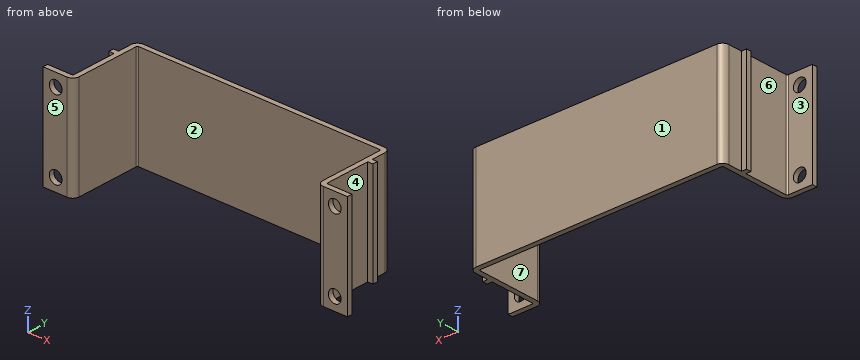
from build123d import *

# Parameters (mm, degrees)
BASE_FLANGE1_DEPTH  = 40
CUT_EXTRUDE1_REACH  = 132
SKETCH6_R           = 2.5
SKETCH7_W           = 2
SKETCH7_H           = 2
BOSS_EXTRUDE1_DEPTH = 40


# Sheet-metal steps are written as plain solids
with BuildPart() as part:
    # Sketch1 → Base-Flange1 (new body)
    with BuildSketch(Plane.XY):
        with BuildLine():
            Line((0, 0), (9.5, 0))
            ThreePointArc((9.5, 0), (9.853553391, 0.146446609), (10, 0.5))
            Line((10, 0.5), (10, 25.5))
            ThreePointArc((10, 25.5), (10.732233047, 27.267766953), (12.5, 28))
            Line((12.5, 28), (107.5, 28))
            ThreePointArc((107.5, 28), (109.267766953, 27.267766953), (110, 25.5))
            Line((110, 25.5), (110, 0.5))
            ThreePointArc((110, 0.5), (110.146446609, 0.146446609), (110.5, 0))
            Line((110.5, 0), (120, 0))
            Line((120, 0), (120, -2))
            Line((120, -2), (110.5, -2))
            ThreePointArc((110.5, -2), (108.732233047, -1.267766953), (108, 0.5))
            Line((108, 0.5), (108, 25.5))
            ThreePointArc((108, 25.5), (107.853553391, 25.853553391), (107.5, 26))
            Line((107.5, 26), (12.5, 26))
            ThreePointArc((12.5, 26), (12.146446609, 25.853553391), (12, 25.5))
            Line((12, 25.5), (12, 0.5))
            ThreePointArc((12, 0.5), (11.267766953, -1.267766953), (9.5, -2))
            Line((9.5, -2), (0, -2))
            Line((0, -2), (0, 0))
        make_face()
    extrude(amount=BASE_FLANGE1_DEPTH)

    # Sketch6 → Cut-Extrude1 (cut, up to next)
    with BuildSketch(Plane.XZ.offset(2), mode=Mode.PRIVATE) as cut_extrude1_sk1:
        with Locations(Location((5, 35, 0), (0, 0, 270))):
            Circle(SKETCH6_R)
    cut_extrude1_tool1 = extrude(cut_extrude1_sk1.sketch, amount=-CUT_EXTRUDE1_REACH, mode=Mode.PRIVATE) & part.part
    # Sketch6 → Cut-Extrude1 (cut, up to next)
    with BuildSketch(Plane.XZ.offset(2), mode=Mode.PRIVATE) as cut_extrude1_sk2:
        with Locations(Location((5, 5, 0), (0, 0, 270))):
            Circle(SKETCH6_R)
    cut_extrude1_tool2 = extrude(cut_extrude1_sk2.sketch, amount=-CUT_EXTRUDE1_REACH, mode=Mode.PRIVATE) & part.part
    # Sketch6 → Cut-Extrude1 (cut, up to next)
    with BuildSketch(Plane.XZ.offset(2), mode=Mode.PRIVATE) as cut_extrude1_sk3:
        with Locations(Location((115, 5, 0), (0, 0, 270))):
            Circle(SKETCH6_R)
    cut_extrude1_tool3 = extrude(cut_extrude1_sk3.sketch, amount=-CUT_EXTRUDE1_REACH, mode=Mode.PRIVATE) & part.part
    # Sketch6 → Cut-Extrude1 (cut, up to next)
    with BuildSketch(Plane.XZ.offset(2), mode=Mode.PRIVATE) as cut_extrude1_sk4:
        with Locations(Location((115, 35, 0), (0, 0, 270))):
            Circle(SKETCH6_R)
    cut_extrude1_tool4 = extrude(cut_extrude1_sk4.sketch, amount=-CUT_EXTRUDE1_REACH, mode=Mode.PRIVATE) & part.part
    add(cut_extrude1_tool1.solids().sort_by_distance((5, -2, 35))[0], mode=Mode.SUBTRACT)
    add(cut_extrude1_tool2.solids().sort_by_distance((5, -2, 5))[0], mode=Mode.SUBTRACT)
    add(cut_extrude1_tool3.solids().sort_by_distance((115, -2, 5))[0], mode=Mode.SUBTRACT)
    add(cut_extrude1_tool4.solids().sort_by_distance((115, -2, 35))[0], mode=Mode.SUBTRACT)

    # Sketch7 → Boss-Extrude1 (add)
    with BuildSketch(Plane.XY.offset(40)):
        with Locations((9, 19)):
            Rectangle(SKETCH7_W, SKETCH7_H)
        with Locations((111, 19)):
            Rectangle(SKETCH7_W, SKETCH7_H)
    extrude(amount=-BOSS_EXTRUDE1_DEPTH)


solid = part.part
Could you check a few things on this model? Use its own coordinates, in mm. Face numbers are marked on the shaded views. A direction names the side the tool comes from. Coordinates: 2 decimals unless noted, no trailing zeros. Write each loop counter-clockwise with the first axis right and the second up, starting at its lowest first coordinate (ties: lowest second). Pieces come first, ordered by that corner, then holes. Notation, with made-up numbers: (-1, 33) - (37, 33) arc R27 cw to (37, 51) - close; hole circle Ø6 at (62, 38.25). An arc over 180 degrees is marked (long way). Write item = value, one per line.
1) For the marked faces 1, 2 and 3, which set-ups out of +Z, -Z, +X, -X, +Y, -Y let a thin tool reach every point of the face, with its end or its side?
Result set:
face_1 = +Z, -Z, +X, -X, +Y
face_2 = +Z, -Z, -Y
face_3 = +Z, -Z, -X
2) Suppose I cut it at C-C on z = 17. Please give me the cut outline in (x, y), plus the area to 3 significant figures.
Result set:
outline = (0, -2) - (9.5, -2) arc R2.5 ccw to (12, 0.5) - (12, 25.5) arc R0.5 cw to (12.5, 26) - (107.5, 26) arc R0.5 cw to (108, 25.5) - (108, 0.5) arc R2.5 ccw to (110.5, -2) - (120, -2) - (120, 0) - (110.5, 0) arc R0.5 cw to (110, 0.5) - (110, 18) - (112, 18) - (112, 20) - (110, 20) - (110, 25.5) arc R2.5 ccw to (107.5, 28) - (12.5, 28) arc R2.5 ccw to (10, 25.5) - (10, 20) - (8, 20) - (8, 18) - (10, 18) - (10, 0.5) arc R0.5 cw to (9.5, 0) - (0, 0) - close
area = 355 mm2
3) We'd pull the mould along Y, two halves only. Please class the marked faces 4, 5, 6 and 7: +Y half, -Y half, draft (parallel to the pull), parting line (faces both ways), or undercut.
Result set:
face_4 = undercut
face_5 = -Y half
face_6 = undercut
face_7 = draft
4) Please list where these lines run through material, in increasing order: line 1 (X direction, y = 3.25, z = 13.5); line 2 (Y direction, x = 58, z = 29); line 3 (Y direction, x = 9, z = 19.5). Write a range as [from, to].
Result set:
line_1 = [10, 12], [108, 110]
line_2 = [26, 28]
line_3 = [-2, 0], [18, 20]
5) Suppose I cut it at A-A on x = 5. Please give me the cut outline in (y, z), plus the area to 3 significant figures.
Result set:
outline = (-2, 0) - (0, 0) - (0, 2.5) - (-2, 2.5) - close; (-2, 7.5) - (0, 7.5) - (0, 32.5) - (-2, 32.5) - close; (-2, 37.5) - (0, 37.5) - (0, 40) - (-2, 40) - close
area = 60.0 mm2
6) Will these pins go through, and if not, where does the flat tip stop? pin 1 Ø12.5 at (y, z) = (18.5, 21) entering from +X; pin 2 Ø1.5 at (y, z) = (11.5, 8.5) entering from +X; pin 3 Ø12 at (x, z) = (64, 21.5) entering from -Y.
Result set:
pin_1 = 112
pin_2 = 110
pin_3 = 26
7) Suppose I cut it at D-D on z = 5. State how many separate pieces and enclosed holes the cut face has, plus the area to 3 significant figures.
Result set:
separate_pieces = 3
enclosed_holes = 0
area = 335 mm2
8) Suppose I cut it at B-B on y = 1.75. Please give me the cut outline in (x, z), plus the area to 3 significant figures.
Result set:
outline = (10, 0) - (12, 0) - (12, 40) - (10, 40) - close; (108, 0) - (110, 0) - (110, 40) - (108, 40) - close
area = 160 mm2
